```python
from build123d import *

# Parameters (mm, degrees)
CYLINDER_R     = 0.75
CYLINDER_DEPTH = 10
BOX_W          = 5
BOX_H          = 15
BOX_DEPTH      = 0.4
FILLET_R       = 2.4


with BuildPart() as cylinder:
    # Cylinder → Cylinder (new body)
    with BuildSketch(Plane(origin=(17.4, 2.4, -4.2), x_dir=(1, 0, 0), z_dir=(0, 0, 1))):
        Circle(CYLINDER_R)
    extrude(amount=CYLINDER_DEPTH)


with BuildPart() as cut:
    # Box → Box (new body)
    with BuildSketch(Plane(origin=(15, 0, 0), x_dir=(1, 0, 0), z_dir=(0, 0, 1))):
        with Locations((2.5, 7.5)):
            Rectangle(BOX_W, BOX_H)
    extrude(amount=BOX_DEPTH)

    # Fillet
    fillet_edges = [cut.edges().sort_by_distance(p)[0] for p in [
        (15, 0, 0.2),
        (20, 0, 0.2),
    ]]
    fillet(fillet_edges, radius=FILLET_R)

    # Cut: cut Cylinder
    add(cylinder.part, mode=Mode.SUBTRACT)


solid = cut.part
```
Part model, mm, in its own coordinate system. Round coordinates to 2 decimals unless told otherwise and drop trailing zeros. Loops run counter-clockwise (first coordinate to the right, second up) from the corner with the lowest first, then second, coordinate; pieces in that order, holes last.
Item 1: Cut at A-A, the plane z = 0.3. Give the cut face in (x, y), then the cut area to 3 significant figures.
Item 2: Drill centre lines: line 1 (X direction, y = 2.4, z = 0.1); line 2 (Y direction, x = 17.4, z = 0.25); line 3 (Y direction, x = 16.3, z = 0.2). Where is each one in solid material? Low to high.
Item 3: Mould opens along Y. For faces 1 (the face through (17, 8, 0)), 2 (the face through (15.684, 0.722, 0.203)), 3 (the face through (18.115, 2.625, 0.197)) say: +Y half, -Y half, draft (parallel to the pull), parting line (faces both ways), or undercut.
Item 4: Cut at B-B, the plane x = 16.9. Give the cut face in (y, z), then the cut area to 3 significant figures.
Item 5: Cut at C-C, the plane x = 18.85. Give the cut face in (y, z).
Item 6: Cut at D-D, the plane x = 16.1. Give the cut face in (y, z), then the cut area to 3 significant figures.
Item 7: Drop a flat-ended pin along its axis: P1, Ø1.7, axis at x = 17.4, y = 2.4, coming from the +Z side. Give the stop position or say it passes through.
A:
1. outline: (15, 2.4) arc R2.4 ccw to (17.4, 0) - (17.6, 0) arc R2.4 ccw to (20, 2.4) - (20, 15) - (15, 15) - close; hole circle Ø1.5 at (17.4, 2.4)
1. area: 70.8 mm2
2. line 1: x = 15 to 16.65, 18.15 to 20
2. line 2: y = 0 to 1.65, 3.15 to 15
2. line 3: y = 0.27 to 15
3. face 1: draft
3. face 2: -Y half
3. face 3: undercut
4. outline: (0.05, 0) - (1.84, 0) - (1.84, 0.4) - (0.05, 0.4) - close; (2.96, 0) - (15, 0) - (15, 0.4) - (2.96, 0.4) - close
4. area: 5.53 mm2
5. outline: (0.35, 0) - (15, 0) - (15, 0.4) - (0.35, 0.4) - close
6. outline: (0.38, 0) - (15, 0) - (15, 0.4) - (0.38, 0.4) - close
6. area: 5.85 mm2
7. P1: stops at z = 0.4
